The figure shows three views and two pictorial views of one solid part (mm, origin at its lowest corner). Answer the questions. A direction names the side the tool comes from. Round coordinates to 2 decimals unless told otherwise and drop trailing zeros. Write each loop counter-clockwise with the first axis right and the second up, starting at its lowest first coordinate (ties: lowest second). Pieces come first, ordered by that corner, then holes. Notation, with made-up numbers: M -20.5,13 L 22.5,13 A19 cw 22.5,45 Z; hole C 77,50 d4. An arc over 180 degrees is marked long. Answer in a Markdown table with one row per item.
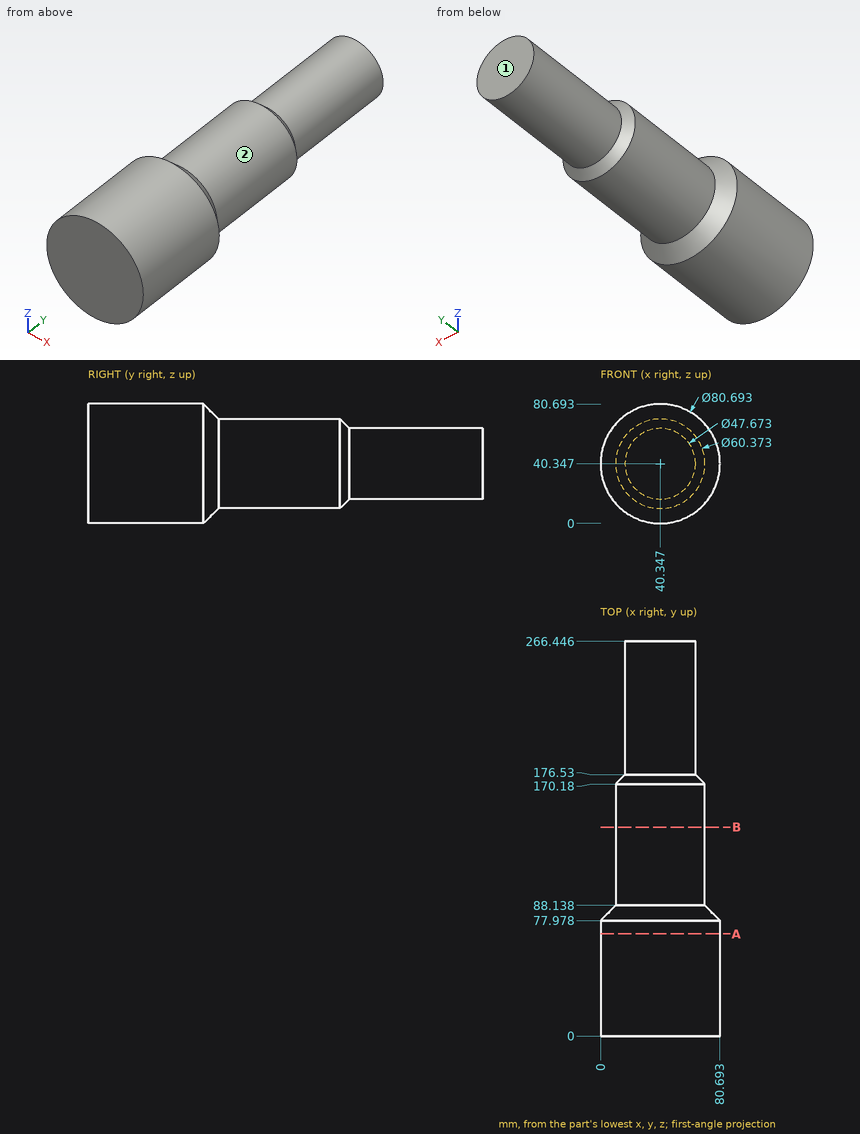
1. A tool of negligible diameter and unlimited length cuts with its end or side. For the marked faces 1 and 2, from which of +Z, -Z, +X, -X, +Y, -Y can it reach the whole face along a straight path? Write none if from no direction.
Calculated:
| item | result |
|---|---|
| face 1 | +Z, -Z, +X, -X, +Y |
| face 2 | +Y |
2. The part is cut by section B-B (y = 141). Determine the outline of the cut face in (x, z).
Calculated:
| item | result |
|---|---|
| outline | C 40.35,40.35 d60.37 |
3. Given pin 1 (4 mm diameter, centred on x = 57, z = 67.5, fed in from +Y); pin 2 (3 mm diameter, centred on x = 63.5, y = 79.5, fed in from -Z); pin 3 (2 mm diameter, centred on y = 100, z = 66.5, fed in from +X) (1 decimal), each flat-ended and moving along its own axis, determine where each tip first touches the part or whether it passes through.
Calculated:
| item | result |
|---|---|
| pin 1 | stops at y = 170.51 |
| pin 2 | stops at z = 7.06 |
| pin 3 | stops at x = 57 |
4. The part is cut by section A-A (y = 69). Determine the outline of the cut face in (x, z), plus the area to 3 significant figures.
Calculated:
| item | result |
|---|---|
| outline | C 40.35,40.35 d80.69 |
| area | 5,110 mm² |
5. Consider line 1 along Y through (x, z) = (69, 12); line 2 along X through (y, z) = (70.5, 19.5); line 3 along Y through (x, z) = (72, 34). Determine where each line is inside the solid, lowest interval first. Write a range as from..to.
Calculated:
| item | result |
|---|---|
| line 1 | y = 0..78.02 |
| line 2 | x = 5.8..74.89 |
| line 3 | y = 0..86.04 |
